The figure shows three views and two pictorial views of one solid part (mm, origin at its lowest corner). Answer the questions. A direction names the side the tool comes from. Round coordinates to 2 decimals unless told otherwise and drop trailing zeros. Order: outer loops, then holes, each group sorted by start corner. A loop starts at its lowest first (then second) coordinate and runs counter-clockwise, first axis right, second up. Notation, with made-up numbers: (37.5, 22.5) - (63.5, 22.5) arc R11 cw to (63.5, 43.5) - close; hole circle Ø2 at (19, 10.25). An arc over 180 degrees is marked (long way). Answer in a Markdown table with one row per item.
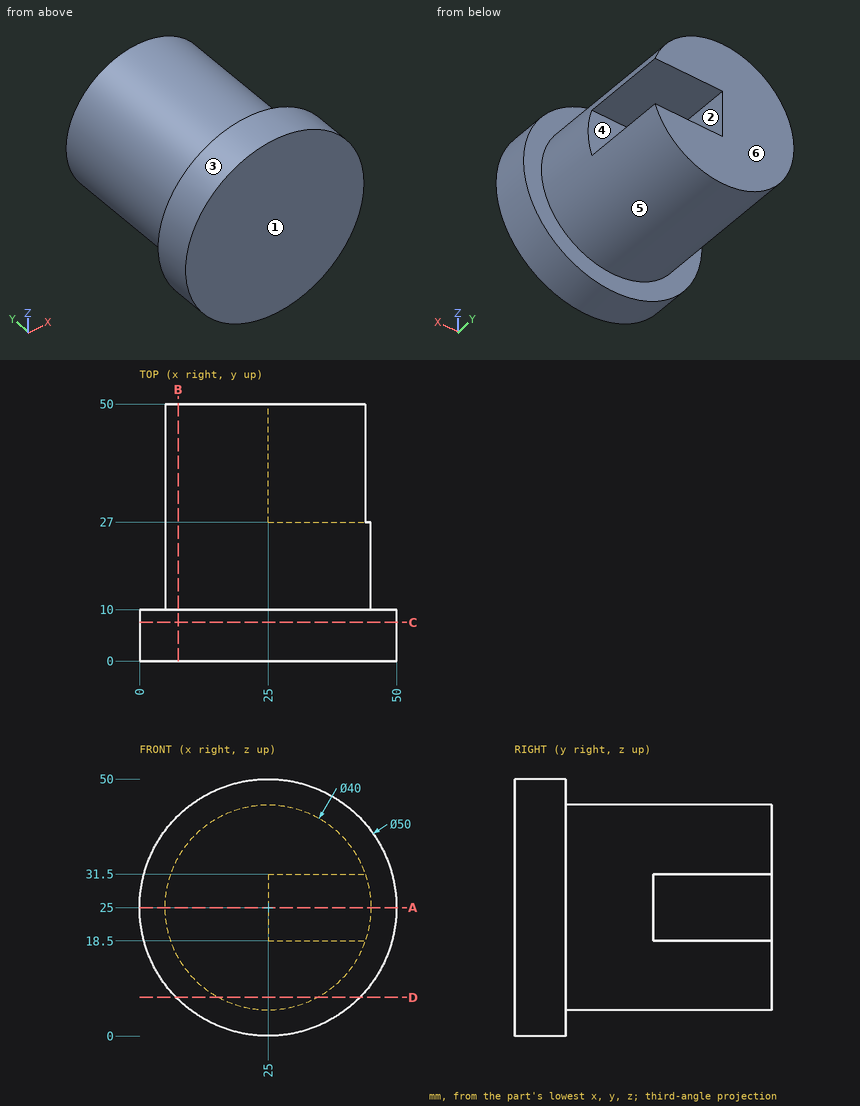
1) Find section B-B, the plane x = 7.5. Give the vertices of the cut face in (y, z).
Filled in:
| item | result |
|---|---|
| outline | (0, 7.15) - (10, 7.15) - (10, 15.32) - (50, 15.32) - (50, 34.68) - (10, 34.68) - (10, 42.85) - (0, 42.85) - close |
2) Find section C-C, the plane y = 7.5. Give the vertices of the cut face in (x, z).
Filled in:
| item | result |
|---|---|
| outline | circle Ø50 at (25, 25) |
3) Find section D-D, the plane z = 7.5. Give the vertices of the cut face in (x, y).
Filled in:
| item | result |
|---|---|
| outline | (7.15, 0) - (42.85, 0) - (42.85, 10) - (34.68, 10) - (34.68, 50) - (15.32, 50) - (15.32, 10) - (7.15, 10) - close |
4) Each of these flat-tipped pins is pushed along its axis until it touches: pin 1 (1.5 mm diameter, centred on x = 9.5, y = 39.5, fed in from -Z); pin 2 (14.5 mm diameter, centred on y = 33.5, z = 28, fed in from +X); pin 3 (3 mm diameter, centred on x = 15.5, y = 19, fed in from -Z). Where does it stop, or does it pass through?
Filled in:
| item | result |
|---|---|
| pin 1 | stops at z = 11.49 |
| pin 2 | stops at x = 45 |
| pin 3 | stops at z = 6.67 |
5) Find the intervals of material crossed by probe 1 along Y at (x, z) = (39.5, 39); probe 2 along Z at (x, y) = (25.5, 16.5); probe 3 along Z at (x, y) = (26, 36), in increasing order. Write a range as from..to.
Filled in:
| item | result |
|---|---|
| probe 1 | y = 0..10 |
| probe 2 | z = 5.01..44.99 |
| probe 3 | z = 5.03..18.5, 31.5..44.97 |
6) Find section A-A, the plane z = 25. Give the vertices of the cut face in (x, y).
Filled in:
| item | result |
|---|---|
| outline | (0, 0) - (50, 0) - (50, 10) - (45, 10) - (45, 27) - (25, 27) - (25, 50) - (5, 50) - (5, 10) - (0, 10) - close |
7) The mould has two halves that part along Z. Classify the marked faces 1, 2 and 3: released by +Z, released by -Z, zero draft, split by the parting line, or undercut.
Filled in:
| item | result |
|---|---|
| face 1 | zero draft |
| face 2 | undercut |
| face 3 | split by the parting line |
8) Which of the six approach directions +Z, -Z, +X, -X, +Y, -Y give full straight-line access (tool end or side, diameter ignored) to the marked faces 4, 5 and 6?
Filled in:
| item | result |
|---|---|
| face 4 | +X, +Y |
| face 5 | +Y |
| face 6 | +Z, -Z, +X, -X, +Y |
